Model file for the job. Use its own axes, mm. Give positions to 0.01 mm unless a question says otherwise; leave off trailing zeros. Write each loop counter-clockwise with the first axis right and the second up, starting at its lowest first coordinate (ties: lowest second). Pieces come first, ordered by that corner, then holes.
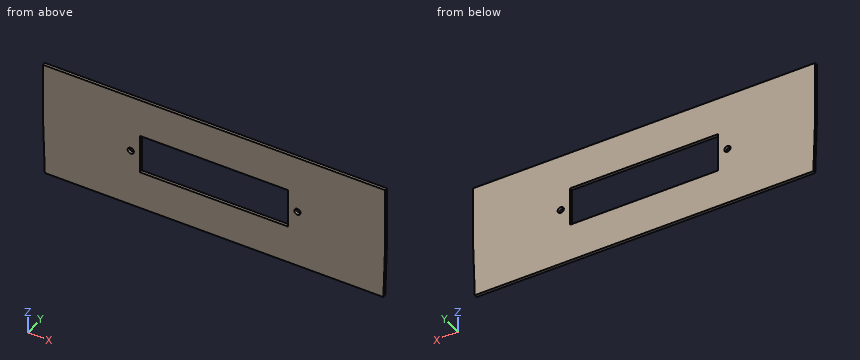
```python
from build123d import *

# Parameters (mm, degrees)
BOSS_EXTRUDE1_DEPTH = 1.7
SKETCH2_R           = 1.75
SKETCH2_W           = 83
SKETCH2_H           = 22
CUT_EXTRUDE1_DEPTH  = 1.7


with BuildPart() as part:
    # Sketch1 → Boss-Extrude1 (new body)
    with BuildSketch(Plane(origin=(0, 0, 0), x_dir=(1, 0, 0), z_dir=(0, 1, 0))):
        Polygon((-96, 0), (-95, 32.5), (95, 32.5), (96, 0), (96, -32.5), (-96, -32.5), align=None)
    extrude(amount=BOSS_EXTRUDE1_DEPTH)

    # Sketch2 → Cut-Extrude1 (cut)
    with BuildSketch(Plane(origin=(0, 1.7, 0), x_dir=(1, 0, 0), z_dir=(0, 1, 0))):
        with Locations((46.75, 0)):
            Circle(SKETCH2_R)
        with Locations((-46.75, 0)):
            Circle(SKETCH2_R)
        Rectangle(SKETCH2_W, SKETCH2_H)
    extrude(amount=-CUT_EXTRUDE1_DEPTH, mode=Mode.SUBTRACT)


solid = part.part
```
1. Slice it at B-B, the plane y = 1.3. Write the cut outline in (x, z), and give its area (3 significant figures).
Calculated:
outline: (-96, 0) - (-95, -32.5) - (95, -32.5) - (96, 0) - (96, 32.5) - (-96, 32.5) - close; hole circle Ø3.5 at (-46.75, 0); hole (-41.5, -11) - (41.5, -11) - (41.5, 11) - (-41.5, 11) - close; hole circle Ø3.5 at (46.75, 0)
area: 10,600 mm2
2. Pin check, flat tip, straight feed: P1, Ø5.5, axis at x = -46.75, z = 0, coming from the +Y side. Stop position of the tip, or through.
Calculated:
P1: stops at y = 1.7
3. Slice it at C-C, the plane z = -3.5. Write the cut outline in (x, y).
Calculated:
outline: (-95.89, 0) - (-41.5, 0) - (-41.5, 1.7) - (-95.89, 1.7) - close; (41.5, 0) - (95.89, 0) - (95.89, 1.7) - (41.5, 1.7) - close
4. Slice it at A-A, the plane x = -46.75. Write the cut outline in (y, z), and give its area (3 significant figures).
Calculated:
outline: (0, -32.5) - (1.7, -32.5) - (1.7, -1.75) - (0, -1.75) - close; (0, 1.75) - (1.7, 1.75) - (1.7, 32.5) - (0, 32.5) - close
area: 105 mm2
5. Probe probe 1 along X at (y, z) = (0.6, 0); probe 2 along Z at (x, y) = (46.75, 0.5); probe 3 along X at (y, z) = (0.1, 4.5). List the from-to ranges inside material, lowest first.
Calculated:
probe 1: x = -96 to -48.5, -45 to -41.5, 41.5 to 45, 48.5 to 96
probe 2: z = -32.5 to -1.75, 1.75 to 32.5
probe 3: x = -96 to -41.5, 41.5 to 96
